For this review, take the finished solid that the model builds, in its own axes (mm). Round coordinates to 2 decimals unless told otherwise and drop trailing zeros. Write each loop counter-clockwise with the first axis right and the second up, starting at its lowest first coordinate (ties: lowest second). Pieces come first, ordered by that corner, then holes. Notation, with made-up numbers: (-30, -26) -> (21, -26) arc R31 cw to (21, 10) -> close; hole circle Ø3 at (54, 7). An arc over 180 degrees is marked (long way). Answer as CSV lines item,"result". Start each with the question number.
Item 1: Take a section at C-C on y = -24.5. Give the boundary of the cut face in (x, z), then the cut area to 3 significant figures.
Item 2: Take a section at B-B on z = 0.25. Give the boundary of the cut face in (x, y).
Item 3: Wall thickness on probe 1 along X at (y, z) = (55.5, 1.2); probe 2 along X at (y, z) = (-4.5, 0.85); probe 3 along Y at (x, z) = (-15, 1.1): over which ranges is each line inside the solid? List them lowest first. Write a range as from..to.
Item 4: Mouldability with a two-part tool opening along Y and no side actions: class faces 1 (the cylindrical face through (55.985, -5.392, 0.789)), 2 (the flat face through (-1, 2, 1.6)), 3 (the cylindrical face through (-34.499, -44.557, 0.789)) as +Y half, -Y half, draft (parallel to the pull), parting line (faces both ways), or undercut.
Item 5: For pin 1 Ø0.5 at (x, z) = (47.5, 0.5) entering from -Y; pin 2 Ø0.8 at (y, z) = (-52, 1) entering from +X (3 decimals), all flat-tipped, find the tip position at first contact; note any pin that passes through.
Item 6: Take a section at A-A on x = 15. Give the boundary of the cut face in (y, z).
```python
from build123d import *

# Parameters (mm, degrees)
SKETCH1_R           = 2.2
BOSS_EXTRUDE1_DEPTH = 1.6


with BuildPart() as part:
    # Sketch1 → Boss-Extrude1 (new body)
    with BuildSketch(Plane.XY):
        with BuildLine():
            Line((-55.362831431, 57.817815724), (-54.172884307, 48.873950258))
            ThreePointArc((-54.172884307, 48.873950258), (-55.355356756, 44.436600749), (-59.329170971, 42.135055108))
            Line((-59.329170971, 42.135055108), (-68.954453082, 40.854448103))
            Line((-68.954453082, 40.854448103), (-67.027453941, 31.788629925))
            Line((-67.027453941, 31.788629925), (-57.601548228, -12.556769902))
            Line((-57.601548228, -12.556769902), (-51.163468122, -42.845555417))
            Line((-51.163468122, -42.845555417), (-38.694980354, -42.845555417))
            ThreePointArc((-38.694980354, -42.845555417), (-34.452339666, -44.60291473), (-32.694980354, -48.845555417))
            Line((-32.694980354, -48.845555417), (-32.694980354, -59.794106668))
            Line((-32.694980354, -59.794106668), (-20, -59.794106668))
            Line((-20, -59.794106668), (0, -59.794106668))
            Line((0, -59.794106668), (20, -59.794106668))
            Line((20, -59.794106668), (32.694980354, -59.794106668))
            Line((32.694980354, -59.794106668), (32.694980354, -48.845555417))
            ThreePointArc((32.694980354, -48.845555417), (34.452339666, -44.60291473), (38.694980354, -42.845555417))
            Line((38.694980354, -42.845555417), (51.163468122, -42.845555417))
            Line((51.163468122, -42.845555417), (57.601548228, -12.556769902))
            Line((57.601548228, -12.556769902), (67.027453941, 31.788629925))
            Line((67.027453941, 31.788629925), (68.954453082, 40.854448103))
            Line((68.954453082, 40.854448103), (59.329170971, 42.135055108))
            ThreePointArc((59.329170971, 42.135055108), (55.355356756, 44.436600749), (54.172884307, 48.873950258))
            Line((54.172884307, 48.873950258), (55.362831431, 57.817815724))
            ThreePointArc((55.362831431, 57.817815724), (27.730985644, 60.303090258), (0, 61.132503503))
            ThreePointArc((0, 61.132503503), (-27.730985644, 60.303090258), (-55.362831431, 57.817815724))
        make_face()
        with Locations((-28.039843587, 56.853282526)):
            Circle(SKETCH1_R, mode=Mode.SUBTRACT)
        with Locations((-54.239442479, -6.730429289)):
            Circle(SKETCH1_R, mode=Mode.SUBTRACT)
        with Locations((-15, -55.294106668)):
            Circle(SKETCH1_R, mode=Mode.SUBTRACT)
        with Locations(Location((15, -55.294106668, 0), (0, 0, 180))):
            Circle(SKETCH1_R, mode=Mode.SUBTRACT)
        with Locations(Location((54.239442479, -6.730429289, 0), (0, 0, 180))):
            Circle(SKETCH1_R, mode=Mode.SUBTRACT)
        with Locations(Location((28.039843587, 56.853282526, 0), (0, 0, 180))):
            Circle(SKETCH1_R, mode=Mode.SUBTRACT)
    extrude(amount=BOSS_EXTRUDE1_DEPTH)


solid = part.part
```
Output values:
1,outline,"(-55.06, 0) -> (55.06, 0) -> (55.06, 1.6) -> (-55.06, 1.6) -> close"
1,area,"176 mm^2"
2,outline,"(-68.95, 40.85) -> (-51.16, -42.85) -> (-38.69, -42.85) arc R6 cw to (-32.69, -48.85) -> (-32.69, -59.79) -> (32.69, -59.79) -> (32.69, -48.85) arc R6 cw to (38.69, -42.85) -> (51.16, -42.85) -> (68.95, 40.85) -> (59.33, 42.14) arc R6 cw to (54.17, 48.87) -> (55.36, 57.82) arc R464 ccw to (-55.36, 57.82) -> (-54.17, 48.87) arc R6 cw to (-59.33, 42.14) -> close; hole circle Ø4.4 at (-54.24, -6.73); hole circle Ø4.4 at (-28.04, 56.85); hole circle Ø4.4 at (-15, -55.29); hole circle Ø4.4 at (15, -55.29); hole circle Ø4.4 at (28.04, 56.85); hole circle Ø4.4 at (54.24, -6.73)"
3,probe 1,"x = -55.05..-29.77, -26.31..26.31, 29.77..55.05"
3,probe 2,"x = -59.31..59.31"
3,probe 3,"y = -59.79..-57.49, -53.09..60.89"
4,face 1,"undercut"
4,face 2,"draft"
4,face 3,"-Y half"
5,pin 1,"stops at y = -42.85"
5,pin 2,"stops at x = 32.695"
6,outline,"(-59.79, 0) -> (-57.49, 0) -> (-57.49, 1.6) -> (-59.79, 1.6) -> close; (-53.09, 0) -> (60.89, 0) -> (60.89, 1.6) -> (-53.09, 1.6) -> close"
